```python
from build123d import *

# Parameters (mm, degrees)
SKETCH1_R           = 9.5
BOSS_EXTRUDE1_DEPTH = 1554
SKETCH2_R           = 3
BOSS_EXTRUDE2_DEPTH = 10
SKETCH3_R           = 3
BOSS_EXTRUDE3_DEPTH = 10


with BuildPart() as part:
    # Sketch1 → Boss-Extrude1 (new body)
    with BuildSketch(Plane(origin=(0, 0, 0), x_dir=(0, 0, -1), z_dir=(1, 0, 0))):
        Circle(SKETCH1_R)
    extrude(amount=BOSS_EXTRUDE1_DEPTH)

    # Sketch2 → Boss-Extrude2 (add)
    with BuildSketch(Plane.ZY):
        Circle(SKETCH2_R)
    extrude(amount=BOSS_EXTRUDE2_DEPTH)

    # Sketch3 → Boss-Extrude3 (add)
    with BuildSketch(Plane(origin=(1554, 0, 0), x_dir=(0, 0, -1), z_dir=(1, 0, 0))):
        Circle(SKETCH3_R)
    extrude(amount=BOSS_EXTRUDE3_DEPTH)


solid = part.part
```
The listing builds one solid part. Answer for the finished solid, in the listing's coordinates (mm). Round coordinates to 2 decimals unless told otherwise and drop trailing zeros. Loops run counter-clockwise (first coordinate to the right, second up) from the corner with the lowest first, then second, coordinate; pieces in that order, holes last.
1) Given P1, Ø8, axis at x = 677, y = 7.5, coming from the -Z side; P2, Ø3, axis at x = 1029, z = 3.5, coming from the +Y side; P3, Ø1.5, axis at y = -5, z = -4.5, coming from the -X side; P4, Ø2, axis at x = 883, y = -0.5, coming from the -Z side, each flat-ended and moving along its own axis, determine where each tip first touches the part or whether it passes through.
Outcome:
P1: stops at z = -8.83
P2: stops at y = 9.29
P3: stops at x = 0
P4: stops at z = -9.5
2) Consider line 1 (X direction, y = -5.75, z = 5.25); line 2 (Y direction, x = 141, z = 1.75); line 3 (Y direction, x = 106.5, z = 0.25). Determine where each line is inside the solid, lowest interval first.
Outcome:
line 1: x = 0 to 1554
line 2: y = -9.34 to 9.34
line 3: y = -9.5 to 9.5
3) A cutting plane is placed at A-A on x = 1169.5. Determine the outline of the cut face in (y, z).
Outcome:
outline: circle Ø19 at (0, 0)
4) A cutting plane is placed at B-B on y = -6. Determine the outline of the cut face in (x, z), plus the area to 3 significant figures.
Outcome:
outline: (0, -7.37) - (1554, -7.37) - (1554, 7.37) - (0, 7.37) - close
area: 22,900 mm2
